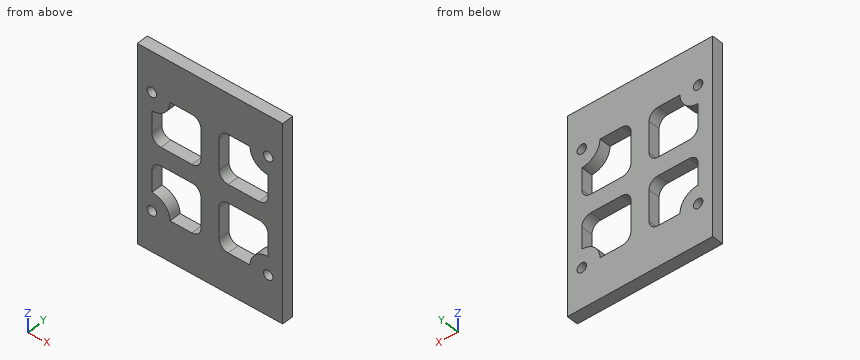
from build123d import *

# Parameters (mm, degrees)
SKETCH1_W           = 80
SKETCH1_H           = 108.18
SKETCH1_R           = 2.6
BOSS_EXTRUDE1_DEPTH = 6.35
CUT_EXTRUDE1_DEPTH  = 6.35


with BuildPart() as part:
    # Sketch1 → Boss-Extrude1 (new body)
    with BuildSketch(Plane(origin=(0, 0, 0), x_dir=(1, 0, 0), z_dir=(0, 1, 0))):
        Rectangle(SKETCH1_W, SKETCH1_H)
        with Locations(Location((-32, 32, 0), (0, 0, 270))):
            Circle(SKETCH1_R, mode=Mode.SUBTRACT)
        with Locations(Location((32, 32, 0), (0, 0, 270))):
            Circle(SKETCH1_R, mode=Mode.SUBTRACT)
        with Locations(Location((32, -32, 0), (0, 0, 270))):
            Circle(SKETCH1_R, mode=Mode.SUBTRACT)
        with Locations(Location((-32, -32, 0), (0, 0, 270))):
            Circle(SKETCH1_R, mode=Mode.SUBTRACT)
    extrude(amount=BOSS_EXTRUDE1_DEPTH)

    # Sketch2 → Cut-Extrude1 (cut)
    with BuildSketch(Plane(origin=(0, 6.35, 0), x_dir=(1, 0, 0), z_dir=(0, 1, 0))):
        with BuildLine():
            Line((-27, -5), (-10, -5))
            ThreePointArc((-10, -5), (-6.464466094, -6.464466094), (-5, -10))
            Line((-5, -10), (-5, -27))
            ThreePointArc((-5, -27), (-6.464466094, -30.535533906), (-10, -32))
            Line((-10, -32), (-22, -32))
            ThreePointArc((-22, -32), (-24.928932188, -24.928932188), (-32, -22))
            Line((-32, -22), (-32, -10))
            ThreePointArc((-32, -10), (-30.535533906, -6.464466094), (-27, -5))
        make_face()
        with BuildLine():
            Line((-22, 32), (-10, 32))
            ThreePointArc((-10, 32), (-6.464466094, 30.535533906), (-5, 27))
            Line((-5, 27), (-5, 10))
            ThreePointArc((-5, 10), (-6.464466094, 6.464466094), (-10, 5))
            Line((-10, 5), (-27, 5))
            ThreePointArc((-27, 5), (-30.535533906, 6.464466094), (-32, 10))
            Line((-32, 10), (-32, 22))
            ThreePointArc((-32, 22), (-24.928932188, 24.928932188), (-22, 32))
        make_face()
        with BuildLine():
            Line((32, 22), (32, 10))
            ThreePointArc((32, 10), (30.535533906, 6.464466094), (27, 5))
            Line((27, 5), (10, 5))
            ThreePointArc((10, 5), (6.464466094, 6.464466094), (5, 10))
            Line((5, 10), (5, 27))
            ThreePointArc((5, 27), (6.464466094, 30.535533906), (10, 32))
            Line((10, 32), (22, 32))
            ThreePointArc((22, 32), (24.928932188, 24.928932188), (32, 22))
        make_face()
        with BuildLine():
            Line((22, -32), (10, -32))
            ThreePointArc((10, -32), (6.464466094, -30.535533906), (5, -27))
            Line((5, -27), (5, -10))
            ThreePointArc((5, -10), (6.464466094, -6.464466094), (10, -5))
            Line((10, -5), (27, -5))
            ThreePointArc((27, -5), (30.535533906, -6.464466094), (32, -10))
            Line((32, -10), (32, -22))
            ThreePointArc((32, -22), (24.928932188, -24.928932188), (22, -32))
        make_face()
    extrude(amount=-CUT_EXTRUDE1_DEPTH, mode=Mode.SUBTRACT)


solid = part.part
The model under review builds one solid part; all positions refer to its coordinate system, in mm. Give positions to 0.01 mm unless a question says otherwise; leave off trailing zeros. Order: outer loops, then holes, each group sorted by start corner. A loop starts at its lowest first (then second) coordinate and runs counter-clockwise, first axis right, second up. Notation, with made-up numbers: M 84,-11 L 94,-11 A31 ccw 94,20 Z; hole C -35.5,-24.75 d10. An arc over 180 degrees is marked long. Answer in a Markdown table with one row per item. Add a question column.
1. To check wall thickness, follow line 1 along Z through (x, y) = (-10, 1.5); line 2 along X through (y, z) = (1.5, -11); line 3 along X through (y, z) = (6, -7). State the ranges of each line that lie inside material, in increasing order.
2. Add section B-B on z = 18. State the section outline as (x, y) points, plus the area to 3 significant figures.
3. Add section C-C on y = 4.75. Count the separate pieces of the cut face and the enclosed holes in it, plus the area to 3 significant figures.
4. Add section A-A on x = 18.5. State the section outline as (y, z) points.
The answers:
| question | item | result |
|---|---|---|
| 1 | line 1 | -54.09 to -32, -5 to 5, 32 to 54.09 |
| 1 | line 2 | -40 to -32, -5 to 5, 32 to 40 |
| 1 | line 3 | -40 to -31, -6 to 6, 31 to 40 |
| 2 | outline | M -40,0 L -32,0 L -32,6.35 L -40,6.35 Z; M -5,0 L 5,0 L 5,6.35 L -5,6.35 Z; M 32,0 L 40,0 L 40,6.35 L 32,6.35 Z |
| 2 | area | 165 mm2 |
| 3 | separate pieces | 1 |
| 3 | enclosed holes | 8 |
| 3 | area | 6,030 mm2 |
| 4 | outline | M 0,-54.09 L 6.35,-54.09 L 6.35,-32 L 0,-32 Z; M 0,-5 L 6.35,-5 L 6.35,5 L 0,5 Z; M 0,32 L 6.35,32 L 6.35,54.09 L 0,54.09 Z |
